Verification items for the finished model (mm, model axes). A direction names the side the tool comes from. Give positions to 0.01 mm unless a question says otherwise; leave off trailing zeros.
(1) Mould release check, pull along X, two halves, no side actions. Record for faces 4 (the face through (10, -6, 39)), 5 (the face through (-2.4, 0.1, 0)), 6 (the face through (2.71, 4.26, 39.44)): pulls with the +X half, pulls with the -X half, needs draft (parallel to the pull), parting line crosses it, or undercut.
(2) Access from +Z, -Z, +X, -X, +Y, -Y to the whole of each face (thin tool, end or side, straight path). Record for faces 1 (the face through (8, 4.15, 39)), 2 (the face through (-2.65, -9, 39)), 3 (the face through (9, 2.65, 39)).
(3) Scan lines: L1, parallel to Y at x = 7, z = 43; L2, parallel to X at y = 6.25, z = 16; L3, parallel to Y at x = 3, z = 13.5. Record each from-to range of solid material in increasing order.
(4) Sectioned sample at A-A on z = 15. Count the separate pieces of the cut face and the enclosed holes in it, plus the area to 3 significant figures.
Autodesk Inventor part; units mm, degrees
ref_plane "YZ Plane" through (0, 0, 0) normal (1, 0, 0) x (0, 1, 0)
ref_plane "XZ Plane" through (0, 0, 0) normal (0, 1, 0) x (-1, 0, 0)
ref_plane "XY Plane" through (0, 0, 0) normal (0, 0, 1) x (1, 0, 0)
sketch "스케치1" plane through (0, 0, 0) normal (0, 0, 1) x (1, 0, 0)
  line L0 (9.7, -10) -> (-9.7, -10)
  line L1 (-10, -9.7) -> (-10, 9.7)
  line L2 (-9.7, 10) -> (9.7, 10)
  line L3 (10, 9.7) -> (10, -9.7)
  line L4 (10, -10) -> (-10, 10) construction
  line L5 (-10, -10) -> (10, 10) construction
  line L6 (7, -7) -> (-7, -7) construction
  line L7 (-7, -7) -> (-7, 7) construction
  line L8 (-7, 7) -> (7, 7) construction
  line L9 (7, 7) -> (7, -7) construction
  line L10 (7, -7) -> (-7, 7) construction
  line L11 (-7, -7) -> (7, 7) construction
  circle A0 centre (-7, 7) radius 2
  circle A1 centre (0, 0) radius 2.15
  arc A2 (9.7, -10) -> (10, -9.7) centre (9.7, -9.7) ccw
  arc A3 (-10, -9.7) -> (-9.7, -10) centre (-9.7, -9.7) ccw
  arc A4 (-9.7, 10) -> (-10, 9.7) centre (-9.7, 9.7) ccw
  arc A5 (10, 9.7) -> (9.7, 10) centre (9.7, 9.7) ccw
  line L12 (0, 10) -> (0, -10) construction
  line L13 (10, 0) -> (-10, 0) construction
  line L14 (2.65, -10) -> (-2.65, -10)
  line L15 (-2.65, -10) -> (-2.65, -8.5)
  line L16 (-2.65, -8.5) -> (2.65, -8.5)
  line L17 (2.65, -8.5) -> (2.65, -10)
  line L18 (4.15, -3.3) -> (-4.15, -3.3) construction
  line L19 (-4.15, -3.3) -> (-4.15, -8.5) construction
  line L20 (-4.15, -8.5) -> (4.15, -8.5)
  line L21 (4.15, -8.5) -> (4.15, -3.3) construction
  arc A6 (4.15, -6.4742) -> (-4.15, -6.4742) centre (0, -7.6) ccw
  line L22 (42.9153, -82.9009) -> (54.7664, -82.9009) construction
  line L23 (54.7664, -82.9009) -> (54.7664, -95.6544) construction
  line L24 (54.7664, -95.6544) -> (42.9153, -95.6544) construction
  line L25 (42.9153, -95.6544) -> (42.9153, -82.9009) construction
  arc A7 (44.9755, -91.1725) -> (50.2986, -91.1614) centre (47.6297, -87.6532) ccw
  line L26 (0, -3.1269) -> (-0.1768, -3.3036)
  line L27 (0, -3.1269) -> (0, -3.3) construction
  line L28 (0, -3.1269) -> (0.1731, -3.1269) construction
  line L29 (47.4573, -92.1078) -> (47.6389, -92.3063)
  line L30 (0, -3.1269) -> (0.1768, -3.3036)
  line L31 (-4.15, -6.4742) -> (-4.15, -8.5)
  line L32 (4.15, -8.5) -> (4.15, -6.4742)
  arc A8 (6.4742, 4.15) -> (6.4742, -4.15) centre (7.6, 0) ccw
  line L33 (8.5, 4.15) -> (6.4742, 4.15)
  line L34 (3.3, -4.15) -> (8.5, -4.15) construction
  line L35 (6.4742, -4.15) -> (8.5, -4.15)
  line L36 (8.5, -4.15) -> (8.5, 4.15)
  line L37 (10, -2.65) -> (8.5, -2.65)
  line L38 (8.5, 2.65) -> (10, 2.65)
  line L39 (3.1269, 0) -> (3.3036, -0.1768)
  line L40 (3.1269, 0) -> (3.3036, 0.1768)
  arc A9 (-4.15, 6.4742) -> (4.15, 6.4742) centre (0, 7.6) ccw
  line L41 (-4.15, 8.5) -> (-4.15, 6.4742)
  line L42 (4.15, 3.3) -> (4.15, 8.5) construction
  line L43 (4.15, 6.4742) -> (4.15, 8.5)
  line L44 (4.15, 8.5) -> (-4.15, 8.5)
  line L45 (2.65, 10) -> (2.65, 8.5)
  line L46 (-2.65, 8.5) -> (-2.65, 10)
  line L47 (0, 3.1269) -> (0.1768, 3.3036)
  line L48 (0, 3.1269) -> (-0.1768, 3.3036)
  arc A10 (-6.4742, -4.15) -> (-6.4742, 4.15) centre (-7.6, 0) ccw
  line L49 (-8.5, -4.15) -> (-6.4742, -4.15)
  line L50 (-3.3, 4.15) -> (-8.5, 4.15) construction
  line L51 (-6.4742, 4.15) -> (-8.5, 4.15)
  line L52 (-8.5, 4.15) -> (-8.5, -4.15)
  line L53 (-10, 2.65) -> (-8.5, 2.65)
  line L54 (-8.5, -2.65) -> (-10, -2.65)
  line L55 (-3.1269, 0) -> (-3.3036, 0.1768)
  line L56 (-3.1269, 0) -> (-3.3036, -0.1768)
  circle A11 centre (-7, -7) radius 2
  circle A12 centre (7, -7) radius 2
  circle A13 centre (7, 7) radius 2
  point P0 (3.3, 0)
  point P1 (0, 3.3)
  point P2 (-3.3, 0)
  point P3 (6.4742, -4.15)
  point P4 (4.15, 6.4742)
  point P5 (-6.4742, 4.15)
  point P6 (-4.15, -6.4742)
  dimension "d0" = 20
  dimension "d1" = 20
  dimension "d2" = 14
  dimension "d3" = 14
  dimension "d4" = 4
  dimension "d5" = 4.3
  dimension "d6" = 0.3
  dimension "d7" = 5.3
  dimension "d8" = 1.5
  dimension "d9" = 6.7
  dimension "d10" = 8.3
  dimension "d11" = 4.3
  dimension "d28" = 0.25
  dimension "d30" = 90
  dimension "d37" = 45
  dimension "d41" = 360
  dimension "d48" = 360
extrude "돌출1" add sketch "스케치1" along normal blind 80 contours L0 L17 L20 L32 A6 L30 L26 L31 L15 A3 L1 L54 L52 L49 A10 L56 L55 L51 L53 A4 L2 L46 L44 L41 A9 L48 L47 L43 L45 A5 L3 L38 L36 L33 A8 L40 L39 L35 L37 A2
properties part number "SAFRS-P-0014"
Ans:
1. face 4: pulls with the +X half
1. face 5: needs draft
1. face 6: undercut
2. face 1: +Z, -Z
2. face 2: +Z, -Z, -Y
2. face 3: +Z, -Z, +X
3. L1: y = -10 to -9, -5 to -4.15, 4.15 to 5, 9 to 10
3. L2: x = -10 to -8.85, -5.15 to -4.08, 4.08 to 5.15, 8.85 to 10
3. L3: y = -10 to -8.5, -4.52 to 4.52, 8.5 to 10
4. separate pieces: 1
4. enclosed holes: 5
4. area: 158 mm2
